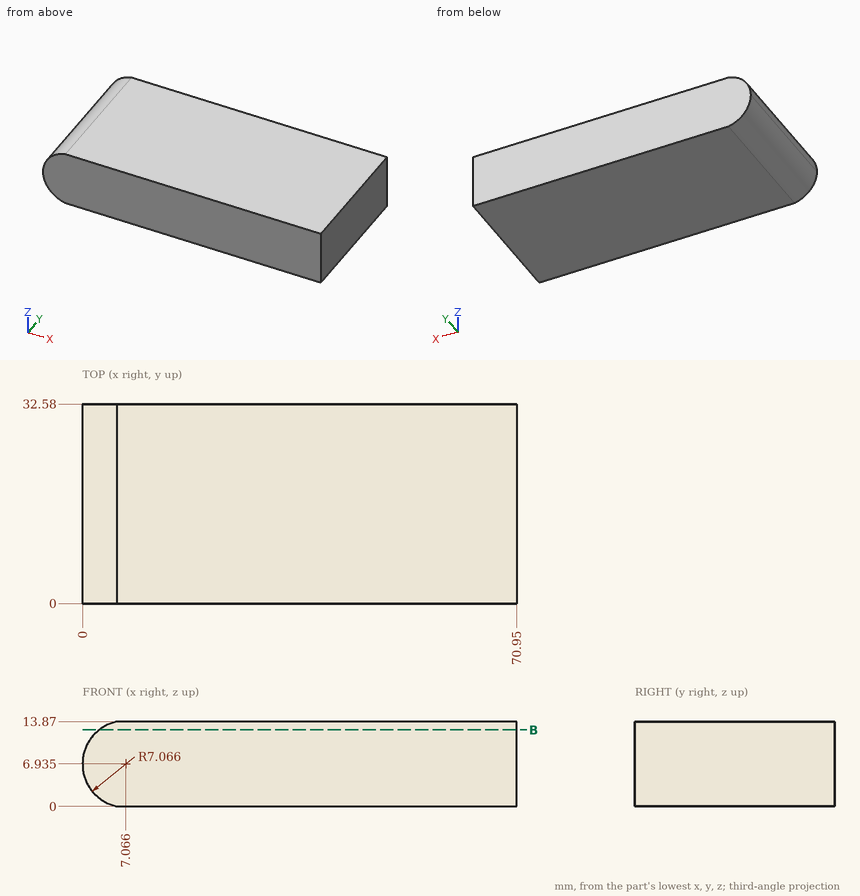
The drawing under review shows one solid part. Ordinate dimensions are in mm from its lowest x, y, z. Coordinates: 2 decimals unless noted, no trailing zeros. Write each loop counter-clockwise with the first axis right and the second up, starting at its lowest first coordinate (ties: lowest second). Pieces come first, ordered by that corner, then holes.
1) To check wall thickness, follow L1, parallel to X at y = 19, z = 12; L2, parallel to X at y = 30, z = 6; L3, parallel to Z at x = 5, y = 13. State the ranges of each line that lie inside material, in increasing order.
2) Insertion check: pin 1 (6 mm diameter, centred on y = 25, z = 11.5, fed in from -X) (1 decimal); pin 2 (4 mm diameter, centred on y = 22, z = 8, fed in from -X). Each pin has a flat end and moves straight along its axis. Give the tip position at first contact, or say it passes through.
3) Add section B-B (z = 12.5). Write out the cut boundary in (x, y), plus the area to 3 significant figures.
Check result:
1. L1: x = 2.14 to 70.95
1. L2: x = 0.06 to 70.95
1. L3: z = 0.18 to 13.69
2. pin 1: stops at x = 0.2
2. pin 2: stops at x = 0
3. outline: (2.71, 0) - (70.95, 0) - (70.95, 32.58) - (2.71, 32.58) - close
3. area: 2,220 mm2
